Check sheet for the modelled part. Datum: model origin and axes. Units: mm. A direction names the side the tool comes from. Coordinates: 2 decimals unless noted, no trailing zeros. Order: outer loops, then holes, each group sorted by start corner. A loop starts at its lowest first (then second) coordinate and runs counter-clockwise, first axis right, second up.
1. Cross-section at B-B (z = 0). Enter the section's corners in (x, y) (3 decimals).
2. Gauge pin test, flat ends, axial feed: pin 1 Ø6.5 at (x, z) = (-0.5, 1.5) entering from -Y; pin 2 Ø5 at (x, z) = (15.5, -15.5) entering from -Y; pin 3 Ø1.2 at (y, z) = (1.5, -26) entering from -X. Record the tip position at first contact, or that the pin passes through.
3. Cross-section at C-C (y = -25.5). Enter the section's corners in (x, z) (3 decimals), then the cut area to 3 significant figures.
4. Thickness scan on line 1 (Y direction, x = 25.5, z = -26); line 2 (X direction, y = 1.95, z = 15.5); line 3 (Z direction, x = -10, y = -28.5) (3 decimals). Record the ranges inside material, lowest first.
5. Draft check along X on faces 1 (the flat face through (-8.5, -29, 26)), 2 (the flat face through (0, -13, -30)), 3 (the flat face through (-16, 2, -26)), 4 (the flat face through (30, -27, -3)). Enter one of: released by +X, released by -X, zero draft, split by the parting line, or undercut.
6. Cross-section at D-D (z = -26). Enter the section's corners in (x, y).
7. Set-up check for faces 5 (the flat face through (0, -17, -21.125)), 6 (the flat face through (0, -24, 26)), 7 (the cylindrical face through (12.57, 6.52, 14.85)), 8 (the flat face through (26, -23, 0)): record each of +Z, -Z, +X, -X, +Y, -Y from which the full face is reachable in a straight line by a thin tool's end or side.
8. Cross-section at A-A (x = -20). Enter the section's corners in (y, z) (3 decimals).
```python
from build123d import *

# Parameters (mm, degrees)
SKETCH1_W           = 60
SKETCH1_H           = 60
BOSS_EXTRUDE1_DEPTH = 8
SKETCH2_R           = 4.5
CUT_EXTRUDE1_DEPTH  = 8
SKETCH3_R           = 11
CUT_EXTRUDE2_DEPTH  = 2.2
SKETCH4_R           = 1.5
CUT_EXTRUDE3_DEPTH  = 11.2
SKETCH6_R           = 3
CUT_EXTRUDE4_DEPTH  = 3
SKETCH7_W           = 60
SKETCH7_H           = 60
SKETCH7_W_2         = 42.25
SKETCH7_H_2         = 42.25
BOSS_EXTRUDE3_DEPTH = 34
SKETCH8_W           = 17
SKETCH8_H           = 8.88
CUT_EXTRUDE5_DEPTH  = 10
SKETCH9_W           = 36
SKETCH9_H           = 20
CUT_EXTRUDE6_DEPTH  = 60
FILLET1_R           = 0.5
FILLET2_R           = 8
FILLET3_R           = 5
SKETCH10_R          = 2
CUT_EXTRUDE7_DEPTH  = 14
CUT_EXTRUDE8_START  = -14
SKETCH11_R          = 2
CUT_EXTRUDE8_DEPTH  = 14


with BuildPart() as part:
    # Sketch1 → Boss-Extrude1 (new body)
    with BuildSketch(Plane(origin=(0, 0, 0), x_dir=(1, 0, 0), z_dir=(0, 1, 0))):
        Rectangle(SKETCH1_W, SKETCH1_H)
    extrude(amount=BOSS_EXTRUDE1_DEPTH)

    # Sketch2 → Cut-Extrude1 (cut)
    with BuildSketch(Plane(origin=(0, 8, 0), x_dir=(1, 0, 0), z_dir=(0, 1, 0))):
        with Locations(Location((0, 0, 0), (0, 0, 270))):
            Circle(SKETCH2_R)
    extrude(amount=-CUT_EXTRUDE1_DEPTH, mode=Mode.SUBTRACT)

    # Sketch3 → Cut-Extrude2 (cut)
    with BuildSketch(Plane.XZ):
        with Locations(Location((0, 0, 0), (0, 0, 270))):
            Circle(SKETCH3_R)
    extrude(amount=-CUT_EXTRUDE2_DEPTH, mode=Mode.SUBTRACT)

    # Sketch4 → Cut-Extrude3 (cut)
    with BuildSketch(Plane.XZ):
        with Locations(Location((-15.5, 15.5, 0), (0, 0, 270))):
            Circle(SKETCH4_R)
        with Locations(Location((-15.5, -15.5, 0), (0, 0, 270))):
            Circle(SKETCH4_R)
        with Locations(Location((15.5, -15.5, 0), (0, 0, 270))):
            Circle(SKETCH4_R)
        with Locations(Location((15.5, 15.5, 0), (0, 0, 270))):
            Circle(SKETCH4_R)
    extrude(amount=-CUT_EXTRUDE3_DEPTH, mode=Mode.SUBTRACT)

    # Sketch6 → Cut-Extrude4 (cut)
    with BuildSketch(Plane(origin=(0, 8, 0), x_dir=(1, 0, 0), z_dir=(0, 1, 0))):
        with Locations(Location((-15.5, 15.5, 0), (0, 0, 270))):
            Circle(SKETCH6_R)
        with Locations(Location((15.5, 15.5, 0), (0, 0, 270))):
            Circle(SKETCH6_R)
        with Locations(Location((-15.5, -15.5, 0), (0, 0, 270))):
            Circle(SKETCH6_R)
        with Locations(Location((15.5, -15.5, 0), (0, 0, 270))):
            Circle(SKETCH6_R)
    extrude(amount=-CUT_EXTRUDE4_DEPTH, mode=Mode.SUBTRACT)

    # Sketch7 → Boss-Extrude3 (add)
    with BuildSketch(Plane.XZ):
        Rectangle(SKETCH7_W, SKETCH7_H)
        Rectangle(SKETCH7_W_2, SKETCH7_H_2, mode=Mode.SUBTRACT)
    extrude(amount=BOSS_EXTRUDE3_DEPTH)

    # Sketch8 → Cut-Extrude5 (cut)
    with BuildSketch(Plane.XZ.offset(34)):
        with Locations((0, 25.56)):
            Rectangle(SKETCH8_W, SKETCH8_H)
    extrude(amount=-CUT_EXTRUDE5_DEPTH, mode=Mode.SUBTRACT)

    # Sketch9 → Cut-Extrude6 (cut)
    with BuildSketch(Plane(origin=(30, 0, 0), x_dir=(0, 0, -1), z_dir=(1, 0, 0))):
        with Locations((0, -13)):
            Rectangle(SKETCH9_W, SKETCH9_H)
    extrude(amount=-CUT_EXTRUDE6_DEPTH, mode=Mode.SUBTRACT)

    # Fillet1
    fillet1_edges = [part.edges().sort_by_distance(p)[0] for p in [
        (0, 8, -4.5),
    ]]
    fillet(fillet1_edges, radius=FILLET1_R)

    # Fillet2
    fillet2_edges = [part.edges().sort_by_distance(p)[0] for p in [
        (-25.5625, -23, 18),
        (-25.5625, -3, 18),
        (-25.5625, -3, -18),
        (-25.5625, -23, -18),
        (25.5625, -23, 18),
        (25.5625, -3, 18),
        (25.5625, -3, -18),
        (25.5625, -23, -18),
    ]]
    fillet(fillet2_edges, radius=FILLET2_R)

    # Fillet3
    fillet3_edges = [part.edges().sort_by_distance(p)[0] for p in [
        (30, -13, 30),
        (-30, -13, 30),
    ]]
    fillet(fillet3_edges, radius=FILLET3_R)

    # Sketch10 → Cut-Extrude7 (cut)
    with BuildSketch(Plane(origin=(30, 0, 0), x_dir=(0, 0, -1), z_dir=(1, 0, 0))):
        with Locations((26, -28.5)):
            Circle(SKETCH10_R)
        with Locations((26, 2.5)):
            Circle(SKETCH10_R)
    extrude(amount=-CUT_EXTRUDE7_DEPTH, mode=Mode.SUBTRACT)

    # Sketch11 → Cut-Extrude8 (cut)
    with BuildSketch(Plane.ZY.offset(30).offset(CUT_EXTRUDE8_START)):
        with Locations(Location((-26, 2.5, 0), (0, 0, 180))):
            Circle(SKETCH11_R)
        with Locations(Location((-26, -28.5, 0), (0, 0, 180))):
            Circle(SKETCH11_R)
    extrude(amount=CUT_EXTRUDE8_DEPTH, mode=Mode.SUBTRACT)


solid = part.part
```
Data:
1. outline: (-30, -34) - (-21.125, -34) - (-21.125, -23) - (-30, -23) - close; (-30, -3) - (-21.125, -3) - (-21.125, 0) - (-11, 0) - (-11, 2.2) - (-4.5, 2.2) - (-4.5, 7.5) arc R0.5 ccw to (-5, 8) - (-30, 8) - close; (4.5, 2.2) - (11, 2.2) - (11, 0) - (21.125, 0) - (21.125, -3) - (30, -3) - (30, 8) - (5, 8) arc R0.5 ccw to (4.5, 7.5) - close; (21.125, -34) - (30, -34) - (30, -23) - (21.125, -23) - close
2. pin 1: stops at y = 2.2
2. pin 2: stops at y = 0
2. pin 3: stops at x = -16
3. outline: (-30, -30) - (30, -30) - (30, 25) arc R5 ccw to (25, 30) - (8.5, 30) - (8.5, 21.125) - (21.125, 21.125) - (21.125, -21.125) - (-21.125, -21.125) - (-21.125, 21.125) - (-8.5, 21.125) - (-8.5, 30) - (-25, 30) arc R5 ccw to (-30, 25) - close
3. area: 1,650 mm2
4. line 1: y = -34 to -30.5, -26.5 to 0.5, 4.5 to 8
4. line 2: x = -30 to -17, -14 to 14, 17 to 30
4. line 3: z = -30 to -21.125, 21.125 to 30
5. face 1: undercut
5. face 2: zero draft
5. face 3: released by -X
5. face 4: released by +X
6. outline: (-30, -34) - (30, -34) - (30, -30.5) - (16, -30.5) - (16, -26.5) - (30, -26.5) - (30, 0.5) - (16, 0.5) - (16, 4.5) - (30, 4.5) - (30, 8) - (-30, 8) - (-30, 4.5) - (-16, 4.5) - (-16, 0.5) - (-30, 0.5) - (-30, -26.5) - (-16, -26.5) - (-16, -30.5) - (-30, -30.5) - close
7. face 5: -Y
7. face 6: +Z, -Y
7. face 7: +Y
7. face 8: +X, -X
8. outline: (-34, -30) - (8, -30) - (8, 30) - (-34, 30) - (-34, 21.125) - (0, 21.125) - (0, -21.125) - (-34, -21.125) - close; hole circle Ø4 at (-28.5, -26); hole circle Ø4 at (2.5, -26)
